Source: CAD feature listing. Evaluate the final solid. Frame: model axes, mm. Face numbers are marked on the shaded views. A direction names the side the tool comes from. Give positions to 0.01 mm unless a question says otherwise; leave off trailing zeros. Order: outer loops, then holes, each group sorted by start corner. A loop starts at its lowest first (then second) coordinate and runs counter-clockwise, first axis right, second up. Notation, with made-up numbers: (61.5, 67.25) - (65.5, 67.25) arc R29 ccw to (65.5, 89.25) - close; hole circle Ø9 at (53.5, -6.5). An arc over 180 degrees is marked (long way). Write each question's results on one line, items separated by ' | '. Start each with the question number.
Item 1: Set-up query: the marked faces 4, 5 and 6. Return all of +Z, -Z, +X, -X, +Y, -Y with unobstructed straight access to the full face (end or side cutting, diameter ignored); none if empty.
Item 2: Section B-B on y = -20.5. Output: boundary loops of the cut face in (x, z), and give its area (3 significant figures).
Item 3: Line query: line 1 along X through (y, z) = (-22, 26); line 2 along Y through (x, z) = (-27.5, 28.5); line 3 along Z through (x, y) = (-23.5, -33). Output: solid intervals per line, ascending.
Item 4: Mould query, pull axis X, two halves, no side actions, for the marked faces 1, 2 and 3. Classes: released by +X, released by -X, zero draft, split by the parting line, or undercut.
Item 5: Contact query for flat-ended pins moving along their axis: pin 1 Ø15 at (x, y) = (-9.5, -30) entering from +Z; pin 2 Ø7.5 at (x, z) = (25.5, 19.5) entering from -Y. Output: stop coordinate, or through.
Item 6: Section C-C on x = 33.5. Output: boundary loops of the cut face in (y, z), and give its area (4 significant figures).
Item 7: Section D-D on x = -2. Output: boundary loops of the cut face in (y, z), and give its area (3 significant figures).
Item 8: Section A-A on z = 19. Output: boundary loops of the cut face in (x, y).
```python
from build123d import *

# Parameters (mm, degrees)
F0_W     = 85
F0_H     = 22
F1_DEPTH = 50
F2_W     = 25
F2_H     = 25
F3_DEPTH = 25
F4_W     = 25
F4_H     = 25
F5_DEPTH = 25


with BuildPart() as f1:
    # F0 (on Front) → F1 (new body)
    with BuildSketch(Plane.XZ):
        Rectangle(F0_W, F0_H)
    extrude(amount=F1_DEPTH)

    # F2 (on face) → F3 (join)
    with BuildSketch(Plane.XY.offset(11)):
        with Locations((30, -12.5)):
            Rectangle(F2_W, F2_H)
    extrude(amount=F3_DEPTH)

    # F4 (on face) → F5 (join)
    with BuildSketch(Plane.XY.offset(11)):
        with Locations((-30, -12.5)):
            Rectangle(F4_W, F4_H)
    extrude(amount=F5_DEPTH)


solid = f1.part
```
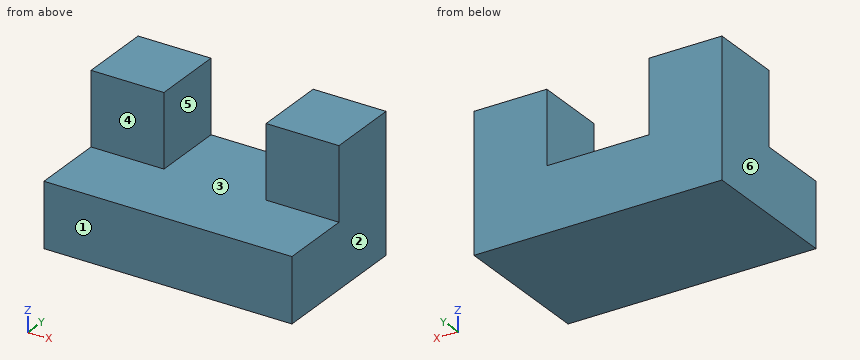
Evaluation:
1) face 4: +Z, +X, -X, -Y | face 5: +Z, +Y, -Y | face 6: +Z, -Z, -X, +Y, -Y
2) outline: (-42.5, -11) - (42.5, -11) - (42.5, 36) - (17.5, 36) - (17.5, 11) - (-17.5, 11) - (-17.5, 36) - (-42.5, 36) - close | area: 3,120 mm^2
3) line 1: x = -42.5 to -17.5, 17.5 to 42.5 | line 2: y = -25 to 0 | line 3: z = -11 to 11
4) face 1: zero draft | face 2: released by +X | face 3: undercut
5) pin 1: stops at z = 11 | pin 2: stops at y = -25
6) outline: (-50, -11) - (0, -11) - (0, 36) - (-25, 36) - (-25, 11) - (-50, 11) - close | area: 1,725 mm^2
7) outline: (-50, -11) - (0, -11) - (0, 11) - (-50, 11) - close | area: 1,100 mm^2
8) outline: (-42.5, -25) - (-17.5, -25) - (-17.5, 0) - (-42.5, 0) - close; (17.5, -25) - (42.5, -25) - (42.5, 0) - (17.5, 0) - close
